Verification items for the finished model (mm, model axes). Face numbers are marked on the shaded views. Round coordinates to 2 decimals unless told otherwise and drop trailing zeros. Order: outer loops, then holes, each group sorted by start corner. A loop starts at its lowest first (then second) coordinate and runs counter-clockwise, first axis right, second up. Notation, with made-up numbers: (3.25, 58.25) -> (45.25, 58.25) arc R28 ccw to (45.25, 82.25) -> close; hole circle Ø8 at (-12, 46). An arc over 180 degrees is marked (long way). Write item = value, one per line. Start each with the question number.
from build123d import *

# Parameters (mm, degrees)
SKETCH1_W                      = 50.8
SKETCH1_H                      = 52.3748
BOSS_EXTRUDE1_DEPTH            = 2.5
F_1_2_0_5_DIAMETER_HOLE1_D     = 12.7
F_3_16_0_1875_DIAMETER_HOLE1_D = 4.7625
FILLET1_R                      = 6.35


with BuildPart() as part:
    # Sketch1 → Boss-Extrude1 (new, symmetric)
    with BuildSketch(Plane.XY):
        Rectangle(SKETCH1_W, SKETCH1_H)
    extrude(amount=BOSS_EXTRUDE1_DEPTH, both=True)

    # 1/2 (0.5) Diameter Hole1 (through all)
    with Locations(Plane.XY.offset(2.5)):
        with Locations((0, -13.4874)):
            Hole(F_1_2_0_5_DIAMETER_HOLE1_D / 2)

    # 3/16 (0.1875) Diameter Hole1 (through all)
    with Locations(Plane(origin=(0, 0, -2.5), x_dir=(-1, 0, 0), z_dir=(0, 0, -1))):
        with Locations((15.5, -6.4874), (7.75, 6.935993759), (-7.75, 6.935993759), (-15.5, -6.4874), (7.75, -19.910793759), (-7.75, -19.910793759)):
            Hole(F_3_16_0_1875_DIAMETER_HOLE1_D / 2)

    # Fillet1
    fillet1_edges = [part.edges().sort_by_distance(p)[0] for p in [
        (25.4, -26.1874, 0),
        (-25.4, -26.1874, 0),
    ]]
    fillet(fillet1_edges, radius=FILLET1_R)


solid = part.part
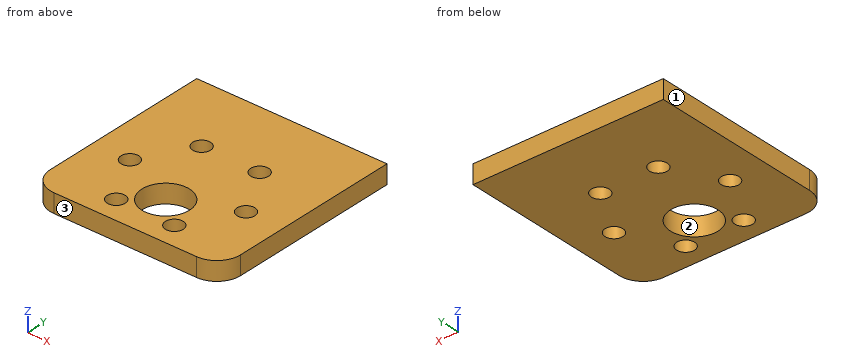
(1) Cross-section at A-A (x = -7.75). Enter the section's corners in (y, z).
(2) Cross-section at B-B (x = 0). Enter the section's corners in (y, z).
(3) Cross-section at C-C (y = -10.5). Enter the section's corners in (x, z).
(4) Draft check along X on the marked faces 1, 2 and 3. Enter one of: +X half, -X half, draft (parallel to the pull), parting line (faces both ways), or undercut.
(5) Cross-section at D-D (z = -1.9). Enter the section's corners in (x, y).
(6) Scan lines: line 1 along Y through (x, z) = (-7.75, 1.05); line 2 along X through (y, z) = (-8, 0.5); line 3 along Y through (x, z) = (15.5, 0.45). Record each from-to range of solid material in increasing order. Write a range as from..to.
Outcome:
q1.outline = (-26.19, -2.5) -> (-22.29, -2.5) -> (-22.29, 2.5) -> (-26.19, 2.5) -> close; (-17.53, -2.5) -> (4.55, -2.5) -> (4.55, 2.5) -> (-17.53, 2.5) -> close; (9.32, -2.5) -> (26.19, -2.5) -> (26.19, 2.5) -> (9.32, 2.5) -> close
q2.outline = (-26.19, -2.5) -> (-19.84, -2.5) -> (-19.84, 2.5) -> (-26.19, 2.5) -> close; (-7.14, -2.5) -> (26.19, -2.5) -> (26.19, 2.5) -> (-7.14, 2.5) -> close
q3.outline = (-25.4, -2.5) -> (-5.6, -2.5) -> (-5.6, 2.5) -> (-25.4, 2.5) -> close; (5.6, -2.5) -> (25.4, -2.5) -> (25.4, 2.5) -> (5.6, 2.5) -> close
q4.face_1 = -X half
q4.face_2 = undercut
q4.face_3 = draft
q5.outline = (-25.4, -19.84) arc R6.35 ccw to (-19.05, -26.19) -> (19.05, -26.19) arc R6.35 ccw to (25.4, -19.84) -> (25.4, 26.19) -> (-25.4, 26.19) -> close; hole circle Ø4.76 at (-15.5, -6.49); hole circle Ø4.76 at (-7.75, -19.91); hole circle Ø4.76 at (-7.75, 6.94); hole circle Ø12.7 at (0, -13.49); hole circle Ø4.76 at (7.75, -19.91); hole circle Ø4.76 at (7.75, 6.94); hole circle Ø4.76 at (15.5, -6.49)
q6.line_1 = -26.19..-22.29, -17.53..4.55, 9.32..26.19
q6.line_2 = -25.4..-17.34, -13.66..-3.2, 3.2..13.66, 17.34..25.4
q6.line_3 = -26.19..-8.87, -4.11..26.19
